from build123d import *

# Parameters (mm, degrees)
CROQUIS1_W              = 110
CROQUIS1_H              = 42
SALIENTE_EXTRUIR1_DEPTH = 30
CHAFL_N1_SIZE           = 10
REDONDEO1_R             = 1
CROQUIS2_R              = 5
CROQUIS2_R_2            = 8
CORTAR_EXTRUIR1_DEPTH   = 30


with BuildPart() as part:
    # Croquis1 → Saliente-Extruir1 (new body)
    with BuildSketch(Plane.XY):
        Rectangle(CROQUIS1_W, CROQUIS1_H)
    extrude(amount=SALIENTE_EXTRUIR1_DEPTH)

    # Chaflán1
    chafl_n1_edges = [part.edges().sort_by_distance(p)[0] for p in [
        (55, -21, 15),
        (-55, -21, 15),
    ]]
    chamfer(chafl_n1_edges, length=CHAFL_N1_SIZE)

    # Redondeo1
    redondeo1_edges = [part.edges().sort_by_distance(p)[0] for p in [
        (-55, 21, 15),
        (55, 21, 15),
    ]]
    fillet(redondeo1_edges, radius=REDONDEO1_R)

    # Croquis2 → Cortar-Extruir1 (cut)
    with BuildSketch(Plane.XY.offset(30)):
        with Locations((-40, -6)):
            Circle(CROQUIS2_R)
        with Locations((40, -6)):
            Circle(CROQUIS2_R)
        with Locations((0, -6)):
            Circle(CROQUIS2_R_2)
    extrude(amount=-CORTAR_EXTRUIR1_DEPTH, mode=Mode.SUBTRACT)


solid = part.part
Can you work these out from the model? Positions are in its coordinate system, mm. Give positions to 0.01 mm unless a question says otherwise; leave off trailing zeros. Order: outer loops, then holes, each group sorted by start corner. A loop starts at its lowest first (then second) coordinate and runs counter-clockwise, first axis right, second up. Notation, with made-up numbers: M 69.25,84 L 79.25,84 A18 cw 79.25,107 Z; hole C 45,-8 d4. An arc over 180 degrees is marked long. One line per question, with ' | ' between items.
Item 1: Suppose I cut it at C-C, the plane z = 23. Write out the boundary of the cut face in (x, y).
Answer block:
outline: M -55,-11 L -45,-21 L 45,-21 L 55,-11 L 55,20 A1 ccw 54,21 L -54,21 A1 ccw -55,20 Z; hole C -40,-6 d10; hole C 0,-6 d16; hole C 40,-6 d10
Item 2: Suppose I cut it at D-D, the plane x = -40. Write out the boundary of the cut face in (y, z).
Answer block:
outline: M -21,0 L -11,0 L -11,30 L -21,30 Z; M -1,0 L 21,0 L 21,30 L -1,30 Z
Item 3: Suppose I cut it at B-B, the plane x = 0. Write out the boundary of the cut face in (y, z), then the cut area to 3 significant figures.
Answer block:
outline: M -21,0 L -14,0 L -14,30 L -21,30 Z; M 2,0 L 21,0 L 21,30 L 2,30 Z | area: 780 mm2
Item 4: Please list where these lines run through material, in increasing order: L1, parallel to Y at x = 40, z = 6.5; L2, parallel to X at y = -7.5, z = 26; L3, parallel to Y at x = 0, z = 12.25.
Answer block:
L1: y = -21 to -11, -1 to 21 | L2: x = -55 to -44.77, -35.23 to -7.86, 7.86 to 35.23, 44.77 to 55 | L3: y = -21 to -14, 2 to 21
Item 5: Suppose I cut it at A-A, the plane y = -6. Write out the boundary of the cut face in (x, z), then the cut area to 3 significant figures.
Answer block:
outline: M -55,0 L -45,0 L -45,30 L -55,30 Z; M -35,0 L -8,0 L -8,30 L -35,30 Z; M 8,0 L 35,0 L 35,30 L 8,30 Z; M 45,0 L 55,0 L 55,30 L 45,30 Z | area: 2,220 mm2
Item 6: I'm going to push flat-ended pins straight in: pin 1 Ø6 at (x, y) = (40, -6) entering from -Z; pin 2 Ø2 at (x, y) = (39, -11) entering from -Z. Where does each tip first touch, or does it pass through?
Answer block:
pin 1: passes through | pin 2: stops at z = 0
